Geometry: final body of the model. Coordinates: model frame, mm. Face numbers are marked on the shaded views. A direction names the side the tool comes from. Coordinates: 2 decimals unless noted, no trailing zeros. Loops run counter-clockwise (first coordinate to the right, second up) from the corner with the lowest first, then second, coordinate; pieces in that order, holes last. Notation, with made-up numbers: (26.25, -24) - (75.25, -24) arc R25 ccw to (75.25, -5) - close; hole circle Ø1 at (18.25, -40). An arc over 180 degrees is marked (long way). Answer in a Markdown table with one row per item.
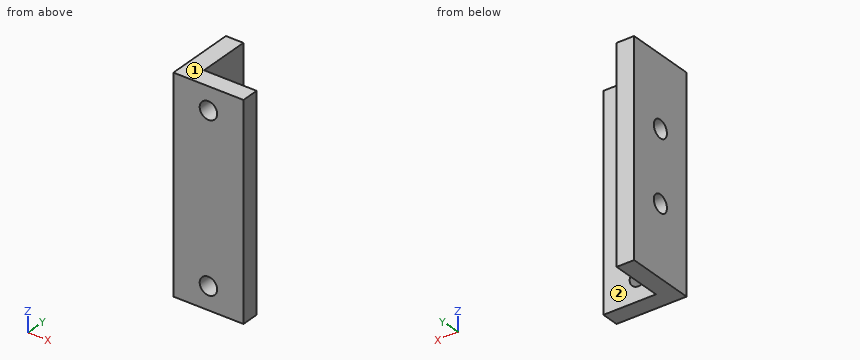
from build123d import *

# Parameters (mm, degrees)
BOSS_EXTRUDE1_DEPTH = 38.1
SKETCH2_R           = 1.5875
CUT_EXTRUDE1_DEPTH  = 43.121134838
SKETCH3_R           = 1.5875
CUT_EXTRUDE2_DEPTH  = 43.121134838


with BuildPart() as part:
    # Sketch1 → Boss-Extrude1 (new body)
    with BuildSketch(Plane.XY):
        Polygon((0, 12.7), (0, 0), (12.7, 0), (12.7, 3.175), (3.175, 3.175), (3.175, 12.7), align=None)
    extrude(amount=BOSS_EXTRUDE1_DEPTH)

    # Sketch2 → Cut-Extrude1 (cut, through all)
    with BuildSketch(Plane.ZY):
        with Locations(Location((12.7, 6.35, 0), (0, 0, 270))):
            Circle(SKETCH2_R)
        with Locations(Location((25.4, 6.35, 0), (0, 0, 270))):
            Circle(SKETCH2_R)
    extrude(amount=-CUT_EXTRUDE1_DEPTH, mode=Mode.SUBTRACT)

    # Sketch3 → Cut-Extrude2 (cut, through all)
    with BuildSketch(Plane.XZ):
        with Locations(Location((6.35, 4.1275, 0), (0, 0, 270))):
            Circle(SKETCH3_R)
        with Locations(Location((6.35, 33.9725, 0), (0, 0, 270))):
            Circle(SKETCH3_R)
    extrude(amount=-CUT_EXTRUDE2_DEPTH, mode=Mode.SUBTRACT)


solid = part.part
(1) Cut plane A-A on y = 6.35. Output: boundary loops of the cut face in (x, z) (1 decimal).
Verdict:
| item | result |
|---|---|
| outline | (0, 0) - (3.2, 0) - (3.2, 11.1) - (0, 11.1) - close; (0, 14.3) - (3.2, 14.3) - (3.2, 23.8) - (0, 23.8) - close; (0, 27) - (3.2, 27) - (3.2, 38.1) - (0, 38.1) - close |
(2) Ray query, probe 1 along Z at (x, y) = (1.2, 6.35); probe 2 along Z at (x, y) = (6.75, 2); probe 3 along Y at (x, z) = (12, 10) (3 decimals). Return the intervals inside material, ascending.
Verdict:
| item | result |
|---|---|
| probe 1 | z = 0 to 11.11, 14.29 to 23.81, 26.99 to 38.1 |
| probe 2 | z = 0 to 2.59, 5.66 to 32.44, 35.51 to 38.1 |
| probe 3 | y = 0 to 3.175 |
(3) First-contact query: pin 1 Ø4 at (x, z) = (6.35, 4.13) entering from +Y (3 decimals); pin 2 Ø1.9 at (y, z) = (6.35, 25.4) entering from -X; pin 3 Ø3 at (y, z) = (9, 26.5) entering from +X (3 decimals). Flat tips, straight axial feed; report the tip coordinate or a pass-through.
Verdict:
| item | result |
|---|---|
| pin 1 | stops at y = 3.175 |
| pin 2 | passes through |
| pin 3 | stops at x = 3.175 |
(4) Cut plane C-C on x = 6.35. Output: boundary loops of the cut face in (y, z) (3 decimals).
Verdict:
| item | result |
|---|---|
| outline | (0, 0) - (3.175, 0) - (3.175, 2.54) - (0, 2.54) - close; (0, 5.715) - (3.175, 5.715) - (3.175, 32.385) - (0, 32.385) - close; (0, 35.56) - (3.175, 35.56) - (3.175, 38.1) - (0, 38.1) - close |
(5) Cut plane D-D on y = 1.5. State how many separate pieces and enclosed holes the cut face has, then the cut area to 3 significant figures.
Verdict:
| item | result |
|---|---|
| separate pieces | 1 |
| enclosed holes | 2 |
| area | 468 mm² |
(6) Cut plane B-B on z = 25.4. Output: boundary loops of the cut face in (x, y) (1 decimal), then the cut area to 3 significant figures.
Verdict:
| item | result |
|---|---|
| outline | (0, 0) - (12.7, 0) - (12.7, 3.2) - (3.2, 3.2) - (3.2, 4.8) - (0, 4.8) - close; (0, 7.9) - (3.2, 7.9) - (3.2, 12.7) - (0, 12.7) - close |
| area | 60.5 mm² |
(7) Access query for the marked faces 1 and 2. Directions: +Z, -Z, +X, -X, +Y, -Y. A direction counts if a zero-diameter tool reaches every point of the face in a straight line with its end or side. Return the directions, or none.
Verdict:
| item | result |
|---|---|
| face 1 | +Z, +X, -X, +Y, -Y |
| face 2 | +Z, -Z, +X, +Y |
